from build123d import *

# Parameters (mm, degrees)
SMUSSO1_SIZE   = 1
SMUSSO2_SIZE   = 2
RACCORDO1_R    = 2
FORO_3_0_3_1_D = 3


with BuildPart() as part:
    # Schizzo1 → Rivoluzione1 (revolve)
    with BuildSketch(Plane(origin=(0, 0, 0), x_dir=(0, 0, -1), z_dir=(1, 0, 0)), mode=Mode.PRIVATE) as rivoluzione1_sk:
        Polygon((-20.837168328, 15), (-20.837168328, 10), (-45.837168328, 10), (-45.837168328, 25), (54.162831672, 25), (54.162831672, 15), (19.162831672, 15), (19.162831672, 18), (14.162831672, 18), (14.162831672, 15), align=None)
    revolve(rivoluzione1_sk.sketch.rotate(Axis((0, 0, 55.346650187), (0, 0, -1)), 90), axis=Axis((0, 0, 55.346650187), (0, 0, -1)))

    # Smusso1
    smusso1_edges = [part.edges().sort_by_distance(p)[0] for p in [
        (-15, 0, -54.162831672),
        (-10, 0, 45.837168328),
    ]]
    chamfer(smusso1_edges, length=SMUSSO1_SIZE)

    # Smusso2
    smusso2_edges = [part.edges().sort_by_distance(p)[0] for p in [
        (-25, 0, 45.837168328),
    ]]
    chamfer(smusso2_edges, length=SMUSSO2_SIZE)

    # Raccordo1
    raccordo1_edges = [part.edges().sort_by_distance(p)[0] for p in [
        (-15, 0, 20.837168328),
    ]]
    fillet(raccordo1_edges, radius=RACCORDO1_R)

    # Foro Ø3.0 (3)-1 (through all)
    with Locations(Plane(origin=(0, -25, 0), x_dir=(-1, 0, 0), z_dir=(0, -1, 0))):
        with Locations((0, -5.837168328)):
            Hole(FORO_3_0_3_1_D / 2)


solid = part.part
Here's how the part is built. I have some questions about the finished solid (model axes, mm). A direction names the side the tool comes from. Coordinates: 2 decimals unless noted, no trailing zeros. Write each loop counter-clockwise with the first axis right and the second up, starting at its lowest first coordinate (ties: lowest second). Pieces come first, ordered by that corner, then holes.
1) If we section it at C-C (z = 27.5): List the corners of the cut face in (x, y) for me, plus the area to 3 significant figures.
Filled in:
outline: circle Ø50 at (0, 0); hole circle Ø20 at (0, 0)
area: 1,650 mm2
2) If we section it at D-D (z = -26.5): List the corners of the cut face in (x, y) for me, plus the area to 3 significant figures.
Filled in:
outline: circle Ø50 at (0, 0); hole circle Ø30 at (0, 0)
area: 1,260 mm2
3) If I drill on line 1 (Z direction, x = 0, y = -17.75); line 2 (Y direction, x = 0, z = 8); line 3 (Y direction, x = -7.5, z = -41.5), over which ranges is the centre line in solid material (lowest first)?
Filled in:
line 1: z = -54.16 to -19.16, -14.16 to 4.34, 7.34 to 45.84
line 2: y = -25 to -15, 15 to 25
line 3: y = -23.85 to -12.99, 12.99 to 23.85
4) If we section it at A-A (y = 0): List the corners of the cut face in (x, z) for me, plus the area to 3 significant figures.
Filled in:
outline: (-25, -54.16) - (-16, -54.16) - (-15, -53.16) - (-15, -19.16) - (-18, -19.16) - (-18, -14.16) - (-15, -14.16) - (-15, 18.84) arc R2 cw to (-13, 20.84) - (-10, 20.84) - (-10, 44.84) - (-11, 45.84) - (-23, 45.84) - (-25, 43.84) - close; (10, 20.84) - (13, 20.84) arc R2 cw to (15, 18.84) - (15, -14.16) - (18, -14.16) - (18, -19.16) - (15, -19.16) - (15, -53.16) - (16, -54.16) - (25, -54.16) - (25, 43.84) - (23, 45.84) - (11, 45.84) - (10, 44.84) - close
area: 2,220 mm2
5) If we section it at B-B (x = 0): Count the separate pieces of the cut face and the enclosed holes in it, plus the area to 3 significant figures.
Filled in:
separate pieces: 4
enclosed holes: 0
area: 2,160 mm2
6) Which directions (+Z, -Z, +X, -X, +Y, -Y) give clear straight access to the entire face, cutting with the end or side of a thin tool? Please do faces 4 (the face through (-4, -15, -14.163)), 5 (the face through (-10, 0, 33)), 6 (the face through (8.06, -12.65, 2.57)).
Filled in:
face 4: none
face 5: +Z, -Z
face 6: -Z
7) Thinking about a two-plate mould opening in Y: for faces 1 (the face through (-13.267, -12.165, -16.628)), 2 (the face through (23.846, -7.509, -5.849)), 3 (the face through (-0.3, 16.3, -54.163)), which applies, +Y half, -Y half, draft (parallel to the pull), parting line (faces both ways), or undercut?
Filled in:
face 1: undercut
face 2: parting line
face 3: draft
8) I'm going to push flat-ended pins straight in: pin 1 (5 mm diameter, centred on y = -13.5, z = 10.5, fed in from -X); pin 2 (4 mm diameter, centred on x = 18, z = 18, fed in from +Y); pin 3 (5 mm diameter, centred on x = 3, y = -7.5, fed in from -Z); pin 4 (2.5 mm diameter, centred on x = 0, z = 5.84, fed in from -Y). Where does each tip first touch, or does it pass through?
Filled in:
pin 1: stops at x = -22.45
pin 2: stops at y = 19.21
pin 3: stops at z = 20.84
pin 4: passes through
